from build123d import *

# Parameters (mm, degrees)
SKIZZE1_R                       = 1.6
SKIZZE1_W                       = 30
SKIZZE1_H                       = 19
AUFSATZ_LINEAR_AUSTRAGEN1_DEPTH = 6


with BuildPart() as part:
    # Skizze1 → Aufsatz-Linear austragen1 (new body)
    with BuildSketch(Plane.XY):
        Polygon((4, 10), (4, 20), (-2, 20), (-2, 30), (4, 30), (4, 40), (-2, 40), (-2, 50), (4, 50), (4, 60), (-2, 60), (-2, 70), (4, 70), (4, 80), (-2, 80), (-2, 90), (4, 90), (4, 100), (-2, 100), (-2, 110), (4, 110), (4, 120), (-2, 120), (-2, 130), (4, 130), (4, 140), (-2, 140), (-2, 150), (4, 150), (4, 160), (-2, 160), (-2, 170), (4, 170), (4, 180), (-2, 180), (-2, 190), (4, 190), (4, 200), (-2, 200), (-2, 210), (4, 210), (4, 220), (34, 250), (44, 250), (44, 256), (54, 256), (54, 250), (64, 250), (64, 256), (74, 256), (74, 250), (84, 250), (84, 256), (94, 256), (94, 250), (104, 250), (104, 256), (114, 256), (114, 250), (124, 250), (124, 256), (134, 256), (134, 250), (144, 250), (144, 256), (154, 256), (154, 250), (164, 250), (164, 256), (174, 256), (174, 250), (184, 250), (184, 256), (194, 256), (194, 250), (204, 250), (204, 256), (214, 256), (214, 250), (224, 250), (224, 256), (234, 256), (234, 250), (244, 250), (244, 256), (254, 256), (254, 250), (264, 250), (264, 256), (274, 256), (274, 250), (304, 220), (304, 210), (310, 210), (310, 200), (304, 200), (304, 190), (310, 190), (310, 180), (304, 180), (304, 170), (310, 170), (310, 160), (304, 160), (304, 150), (310, 150), (310, 140), (304, 140), (304, 130), (310, 130), (310, 120), (304, 120), (304, 110), (310, 110), (310, 100), (304, 100), (304, 90), (310, 90), (310, 80), (304, 80), (304, 70), (310, 70), (310, 60), (304, 60), (304, 50), (310, 50), (310, 40), (304, 40), (304, 30), (310, 30), (310, 20), (304, 20), (304, 10), (310, 10), (310, 0), (304, 0), (4, 0), (-2, 0), (-2, 10), align=None)
        with Locations((20, 215)):
            Circle(SKIZZE1_R, mode=Mode.SUBTRACT)
        with Locations((30, 215)):
            Circle(SKIZZE1_R, mode=Mode.SUBTRACT)
        with Locations((290, 215)):
            Circle(SKIZZE1_R, mode=Mode.SUBTRACT)
        with Locations((280, 215)):
            Circle(SKIZZE1_R, mode=Mode.SUBTRACT)
        with Locations((20, 36)):
            Circle(SKIZZE1_R, mode=Mode.SUBTRACT)
        with Locations((155, 36)):
            Circle(SKIZZE1_R, mode=Mode.SUBTRACT)
        with Locations((290, 36)):
            Circle(SKIZZE1_R, mode=Mode.SUBTRACT)
        with Locations((260, 30.5)):
            Rectangle(SKIZZE1_W, SKIZZE1_H, mode=Mode.SUBTRACT)
    extrude(amount=AUFSATZ_LINEAR_AUSTRAGEN1_DEPTH)


solid = part.part
Geometry check sheet. Reference: the model listing, model coordinates, mm. Give positions to 0.01 mm unless a question says otherwise; leave off trailing zeros. Order: outer loops, then holes, each group sorted by start corner. A loop starts at its lowest first (then second) coordinate and runs counter-clockwise, first axis right, second up.
1) Cross-section at A-A (z = 1.8). Give the number of separate pieces and of enclosed holes in the cut face, then the cut area to 3 significant figures.
Results are:
separate pieces: 1
enclosed holes: 8
area: 75,500 mm2
2) Gauge pin test, flat ends, axial feed: pin 1 (1.8 mm diameter, centred on y = 253, z = 3.5, fed in from -X); pin 2 (2 mm diameter, centred on y = 222.5, z = 1.5, fed in from -X); pin 3 (3 mm diameter, centred on x = 308, z = 1.5, fed in from -Y); pin 4 (3 mm diameter, centred on y = 75, z = 1, fed in from +X). Record the tip position at first contact, or that the pin passes through.
Results are:
pin 1: stops at x = 44
pin 2: stops at x = 5.5
pin 3: stops at y = 0
pin 4: stops at x = 304
3) Cross-section at B-B (x = 58). Record the boundary of the cut face in (y, z).
Results are:
outline: (0, 0) - (250, 0) - (250, 6) - (0, 6) - close
4) Material ranges on probe 1 along Y at (x, z) = (290, 3.9); probe 2 along X at (y, z) = (215, 3.1); probe 3 along Y at (x, z) = (155, 1.25), recorded low to high.
Results are:
probe 1: y = 0 to 34.4, 37.6 to 213.4, 216.6 to 234
probe 2: x = 4 to 18.4, 21.6 to 28.4, 31.6 to 278.4, 281.6 to 288.4, 291.6 to 304
probe 3: y = 0 to 34.4, 37.6 to 250
